```python
from build123d import *

# Parameters (mm, degrees)
F2_DEPTH = 3.175
F5_DEPTH = 101.6


with BuildPart() as f2:
    # F1 (on offset) → F2 (new body)
    with BuildSketch(Plane.YZ.offset(50.8)):
        Polygon((-68.286333, 76.2), (-134.548811, 0), (79.343306, 0), (79.343306, 76.2), align=None)
    extrude(amount=F2_DEPTH)



with BuildPart() as f3_1:
    # F3: instance of F2
    add(f2.part.mirror(Plane.YZ))


with BuildPart() as f2_1:
    add(f2.part)

    add(f3_1.part)  # F5 merges F3_1
    # F4 (on face) → F5 (join, through all)
    with BuildSketch(Plane(origin=(50.8, 0, 0), x_dir=(0, -1, 0), z_dir=(-1, 0, 0))):
        Polygon((68.286333, 76.2), (-79.343306, 76.2), (-79.343306, 73.025), (71.047269, 73.025), align=None)
    extrude(amount=F5_DEPTH)


solid = f2_1.part
```
Check sheet for the modelled part. Datum: model origin and axes. Units: mm. A direction names the side the tool comes from. Give positions to 0.01 mm unless a question says otherwise; leave off trailing zeros. Order: outer loops, then holes, each group sorted by start corner. A loop starts at its lowest first (then second) coordinate and runs counter-clockwise, first axis right, second up. Notation, with made-up numbers: M 31,12 L 41,12 A30 ccw 41,40 Z; hole C 79.25,68.5 d10. An arc over 180 degrees is marked long. Answer in a Markdown table with one row per item. Add a question column.
Q1. Access from +Z, -Z, +X, -X, +Y, -Y to the whole of each face (thin tool, end or side, straight path). Record for faces 1 (the flat face through (1, 5, 73.025)), 2 (the flat face through (1, 4, 76.2)).
Q2. Gauge pin test, flat end, axial feed: pin 1 Ø8 at (x, y) = (5, -69) entering from -Z (3 decimals). Record the tip position at first contact, or that the pin passes through.
Q3. Sectioned sample at A-A, the plane y = 65. Record the boundary of the cut face in (x, z) (3 decimals).
Q4. Release check for a two-part mould opening along X. For faces 3 (the flat face through (-53.975, -5, 39)), 4 (the flat face through (-52.365, -100.954, 38.633)), 5 (the flat face through (-50.8, -5, 39)) record: released by +X, released by -X, zero draft, split by the parting line, or undercut.
Q5. Sectioned sample at B-B, the plane z = 14. Record the boundary of the cut face in (x, y) (3 decimals), and give its area (3 significant figures).
Q6. Sectioned sample at C-C, the plane z = 41.5. Record the boundary of the cut face in (x, y) (3 decimals).
Q7. Sectioned sample at D-D, the plane x = 26. Record the boundary of the cut face in (y, z) (3 decimals).
Q8. Thickness scan on L1, parallel to X at y = 50, z = 66.5 (3 decimals); L2, parallel to Z at x = -16, y = 33.5 (3 decimals). Record the ranges inside material, lowest first.
Verdict:
| question | item | result |
|---|---|---|
| 1 | face 1 | -Z, +Y, -Y |
| 1 | face 2 | +Z, +X, -X, +Y, -Y |
| 2 | pin 1 | z = 73.025 |
| 3 | outline | M -53.975,0 L -50.8,0 L -50.8,73.025 L 50.8,73.025 L 50.8,0 L 53.975,0 L 53.975,76.2 L -53.975,76.2 Z |
| 4 | face 3 | released by -X |
| 4 | face 4 | zero draft |
| 4 | face 5 | undercut |
| 5 | outline | M -53.975,-122.375 L -50.8,-122.375 L -50.8,79.343 L -53.975,79.343 Z; M 50.8,-122.375 L 53.975,-122.375 L 53.975,79.343 L 50.8,79.343 Z |
| 5 | area | 1,280 mm² |
| 6 | outline | M -53.975,-98.461 L -50.8,-98.461 L -50.8,79.343 L -53.975,79.343 Z; M 50.8,-98.461 L 53.975,-98.461 L 53.975,79.343 L 50.8,79.343 Z |
| 7 | outline | M -71.047,73.025 L 79.343,73.025 L 79.343,76.2 L -68.286,76.2 Z |
| 8 | L1 | -53.975 to -50.8, 50.8 to 53.975 |
| 8 | L2 | 73.025 to 76.2 |
